The figure shows three views and two pictorial views of one solid part (mm, origin at its lowest corner). Answer the questions. A direction names the side the tool comes from. Round coordinates to 2 decimals unless told otherwise and drop trailing zeros. Order: outer loops, then holes, each group sorted by start corner. A loop starts at its lowest first (then second) coordinate and runs counter-clockwise, first axis right, second up.
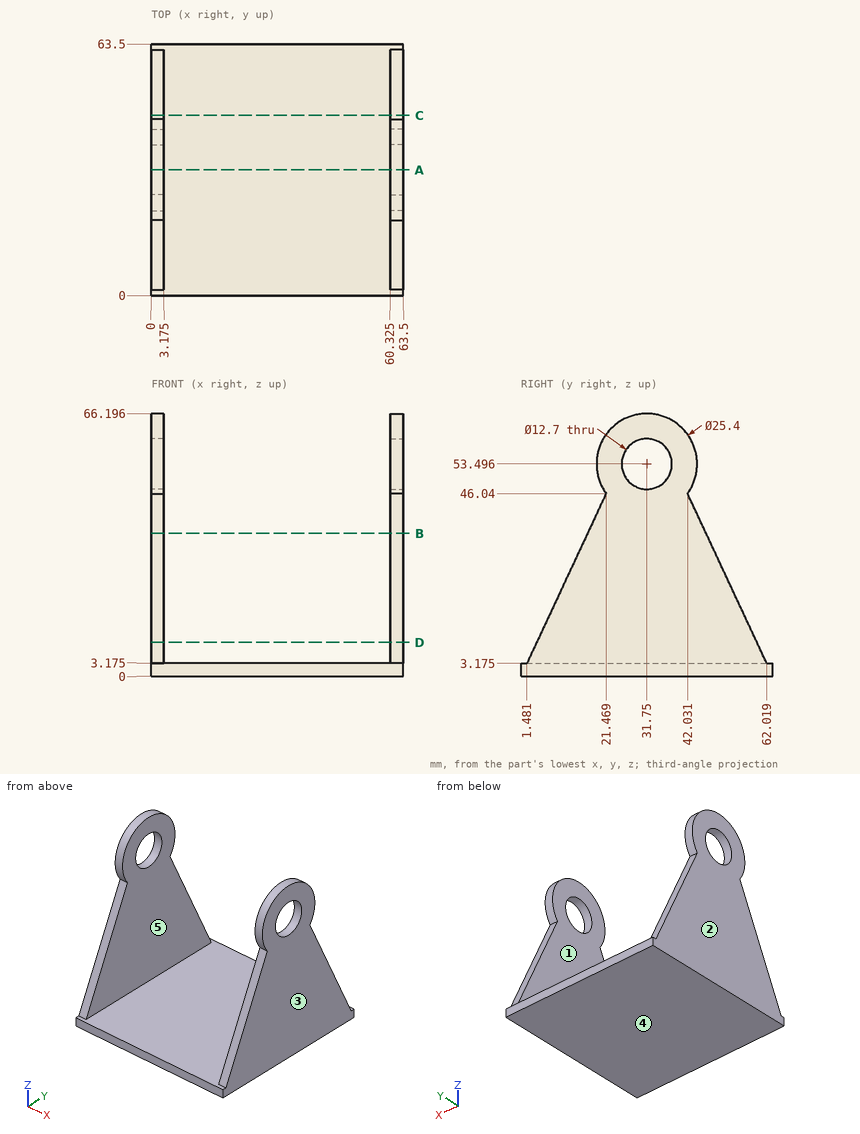
Item 1: Given pin 1 (4 mm diameter, centred on x = 30, y = 17.5, fed in from +Z) (3 decimals), flat-ended and moving along its own axis, determine where the tip first touches the part or whether it passes through.
Item 2: Find the intervals of material crossed by line 1 along Z through (x, y) = (62.1, 31.75); line 2 along X through (y, z) = (35, 61) (1 decimal); line 3 along Z through (x, y) = (31, 36) (1 decimal), in increasing order.
Item 3: For a pull along X with two mould halves and no side action, classify the marked faces 3, 4 and 5 as released by +X, released by -X, zero draft, split by the parting line, or undercut.
Item 4: Find section D-D (z = 8.5). Write down the section's boundary in (x, y) (1 decimal).
Item 5: Find section C-C (y = 45.5). Write down the section's boundary in (x, z) (1 decimal).
Item 6: Find section B-B (z = 36). Write down the section's boundary in (x, y) (1 decimal).
Item 7: A tool of negligible diameter and unlimited length cuts with its end or side. For the marked faces 1 and 2, from which of +Z, -Z, +X, -X, +Y, -Y can it reach the whole face along a straight path? Write none if from no direction.
Item 8: Find section A-A (y = 31.75). Write down the section's boundary in (x, z) (1 decimal).
Model answer:
1. pin 1: stops at z = 3.175
2. line 1: z = 0 to 47.15, 59.85 to 66.2
2. line 2: x = 0 to 3.2, 60.3 to 63.5
2. line 3: z = 0 to 3.2
3. face 3: released by +X
3. face 4: zero draft
3. face 5: undercut
4. outline: (0, 4) - (3.2, 4) - (3.2, 59.5) - (0, 59.5) - close; (60.3, 4) - (63.5, 4) - (63.5, 59.5) - (60.3, 59.5) - close
5. outline: (0, 0) - (63.5, 0) - (63.5, 38.6) - (60.3, 38.6) - (60.3, 3.2) - (3.2, 3.2) - (3.2, 38.6) - (0, 38.6) - close
6. outline: (0, 16.8) - (3.2, 16.8) - (3.2, 46.7) - (0, 46.7) - close; (60.3, 16.8) - (63.5, 16.8) - (63.5, 46.7) - (60.3, 46.7) - close
7. face 1: +Z, +Y, -Y
7. face 2: +Z, -Z, -X, +Y, -Y
8. outline: (0, 0) - (63.5, 0) - (63.5, 47.1) - (60.3, 47.1) - (60.3, 3.2) - (3.2, 3.2) - (3.2, 47.1) - (0, 47.1) - close; (0, 59.8) - (3.2, 59.8) - (3.2, 66.2) - (0, 66.2) - close; (60.3, 59.8) - (63.5, 59.8) - (63.5, 66.2) - (60.3, 66.2) - close
